Check sheet for the modelled part. Datum: model origin and axes. Units: mm. A direction names the side the tool comes from. Round coordinates to 2 decimals unless told otherwise and drop trailing zeros. Write each loop counter-clockwise with the first axis right and the second up, starting at its lowest first coordinate (ties: lowest second). Pieces come first, ordered by that corner, then holes. Notation, with made-up numbers: (59.5, 59) -> (64.5, 59) arc R29 ccw to (64.5, 86) -> close; hole circle Ø9 at (46, -7). An arc over 180 degrees is marked (long way). Use one line per item in the form item = value. Start each with the question number.
```python
from build123d import *

# Parameters (mm, degrees)
SKETCH1_W               = 19
SKETCH1_H               = 16
BOSS_EXTRUDE1_DEPTH     = 30
SKETCH2_R               = 3.5
BOSS_EXTRUDE2_DEPTH     = 26
SKETCH3_R               = 2.5
BOSS_EXTRUDE3_DEPTH     = 6
SKETCH4_R               = 1
CUT_EXTRUDE2_DEPTH      = 60.674114991
SKETCH5_R               = 3.5
SKETCH5_R_2             = 2.5
CUT_EXTRUDE3_DEPTH      = 16
CUT_EXTRUDE4_DEPTH      = 58.36070093
CUT_EXTRUDE4_DEPTH_BACK = 58.36070093
SKETCH6_W               = 2.5
SKETCH6_H               = 8


with BuildPart() as part:
    # Sketch1 → Boss-Extrude1 (new body)
    with BuildSketch(Plane(origin=(0, 0, 0), x_dir=(1, 0, 0), z_dir=(0, 1, 0))):
        Rectangle(SKETCH1_W, SKETCH1_H)
    extrude(amount=BOSS_EXTRUDE1_DEPTH)

    # Sketch2 → Boss-Extrude2 (add)
    with BuildSketch(Plane(origin=(0, 30, 0), x_dir=(1, 0, 0), z_dir=(0, 1, 0))):
        with Locations(Location((0, 0, 0), (0, 0, 90))):
            Circle(SKETCH2_R)
    extrude(amount=BOSS_EXTRUDE2_DEPTH)

    # Sketch3 → Boss-Extrude3 (add)
    with BuildSketch(Plane.XZ):
        with Locations(Location((0, 0, 0), (0, 0, 270))):
            Circle(SKETCH3_R)
    extrude(amount=BOSS_EXTRUDE3_DEPTH)

    # Sketch4 → Cut-Extrude2 (cut, through all)
    with BuildSketch(Plane(origin=(9.5, 0, 0), x_dir=(0, 0, -1), z_dir=(1, 0, 0))):
        with Locations((0, 54)):
            Circle(SKETCH4_R)
    extrude(amount=-CUT_EXTRUDE2_DEPTH, mode=Mode.SUBTRACT)

    # Sketch5 → Cut-Extrude3 (cut)
    with BuildSketch(Plane(origin=(0, 30, 0), x_dir=(1, 0, 0), z_dir=(0, 1, 0))):
        with Locations(Location((0, 0, 0), (0, 0, 270))):
            Circle(SKETCH5_R)
        with Locations(Location((0, 0, 0), (0, 0, 90))):
            Circle(SKETCH5_R_2, mode=Mode.SUBTRACT)
    extrude(amount=CUT_EXTRUDE3_DEPTH, mode=Mode.SUBTRACT)

    # Sketch6 → Cut-Extrude4 (cut, two sides: drawn at the far end of the back side and taken through both)
    with BuildSketch(Plane.XY.offset(-CUT_EXTRUDE4_DEPTH_BACK)):
        with Locations((0, 52)):
            Rectangle(SKETCH6_W, SKETCH6_H)
    extrude(amount=CUT_EXTRUDE4_DEPTH + CUT_EXTRUDE4_DEPTH_BACK, mode=Mode.SUBTRACT)


solid = part.part
```
1. Sectioned sample at D-D (z = 5). Enter the section's corners in (x, y), and give its area (3 significant figures).
2. Depth check by flat-ended pin: pin 1 (0.8 mm diameter, centred on x = 0, z = 1, fed in from +Y); pin 2 (7 mm diameter, centred on y = 53, z = -1, fed in from -X); pin 3 (3 mm diameter, centred on x = -7, z = -4.5, fed in from -Y). Enter the tip coordinate at first touch or a pass-through.
3. Scan lines: probe 1 along Y at (x, z) = (2.9, 0); probe 2 along Y at (x, z) = (2.25, 0); probe 3 along Y at (x, z) = (-1.75, 2.25). Record each from-to range of solid material in increasing order.
4. Sectioned sample at A-A (z = 0). Enter the section's corners in (x, y).
5. Tool access check on faces 1 (the face through (-1.25, 52, 0)), 2 (the face through (2.44, 37.89, 0.54)), 3 (the face through (2, 54, 1)), 4 (the face through (-2, 0, -2)). Record the directions out of +Z, -Z, +X, -X, +Y, -Y that give a thin tool (end or side, any length) a straight path to the whole face; none if there is none.
6. Mould release check, pull along X, two halves, no side actions. Record for faces 5 (the face through (0, -6, 0)), 6 (the face through (3.105, 50.93, -1.615)), 7 (the face through (1.25, 52, 0)): +X half, -X half, draft (parallel to the pull), parting line (faces both ways), or undercut.
7. Sectioned sample at B-B (y = 54). Enter the section's corners in (x, z).
8. Sectioned sample at C-C (x = -5.75). Enter the section's corners in (y, z), and give its area (3 significant figures).
Returned:
q1.outline = (-9.5, 0) -> (9.5, 0) -> (9.5, 30) -> (-9.5, 30) -> close
q1.area = 570 mm^2
q2.pin_1 = 48
q2.pin_2 = -3.5
q2.pin_3 = 0
q3.probe_1 = 0 to 30, 46 to 53, 55 to 56
q3.probe_2 = -6 to 53, 55 to 56
q3.probe_3 = 0 to 30, 46 to 56
q4.outline = (-9.5, 0) -> (-2.5, 0) -> (-2.5, -6) -> (2.5, -6) -> (2.5, 0) -> (9.5, 0) -> (9.5, 30) -> (2.5, 30) -> (2.5, 46) -> (3.5, 46) -> (3.5, 53) -> (1.25, 53) -> (1.25, 48) -> (-1.25, 48) -> (-1.25, 53) -> (-3.5, 53) -> (-3.5, 46) -> (-2.5, 46) -> (-2.5, 30) -> (-9.5, 30) -> close; (-3.5, 55) -> (-1.25, 55) -> (-1.25, 56) -> (-3.5, 56) -> close; (1.25, 55) -> (3.5, 55) -> (3.5, 56) -> (1.25, 56) -> close
q5.face_1 = +Z, -Z, +Y
q5.face_2 = none
q5.face_3 = +X, -X
q5.face_4 = -Y
q6.face_5 = draft
q6.face_6 = parting line
q6.face_7 = undercut
q7.outline = (-3.35, -1) arc R3.5 ccw to (-1.25, -3.27) -> (-1.25, -1) -> close; (-3.35, 1) -> (-1.25, 1) -> (-1.25, 3.27) arc R3.5 ccw to start; (1.25, -3.27) arc R3.5 ccw to (3.35, -1) -> (1.25, -1) -> close; (1.25, 1) -> (3.35, 1) arc R3.5 ccw to (1.25, 3.27) -> close
q8.outline = (0, -8) -> (30, -8) -> (30, 8) -> (0, 8) -> close
q8.area = 480 mm^2
